Design review of the part built by this model. Coordinates are the model's own, in mm. Coordinates: 2 decimals unless noted, no trailing zeros. Order: outer loops, then holes, each group sorted by start corner. A loop starts at its lowest first (then second) coordinate and runs counter-clockwise, first axis right, second up. Notation, with made-up numbers: M -11.5,-9.5 L 4.5,-9.5 A18 cw 4.5,12.5 Z; hole C 6,84.25 d9. An arc over 180 degrees is marked long. Answer as a JSON object with one key per item and string values.
from build123d import *

# Parameters (mm, degrees)
SKETCH_1_R      = 12.5
SKETCH_1_R_2    = 2.1
SKETCH_1_R_3    = 1.6
EXTRUDE_1_DEPTH = 3
FILLET_2_R      = 7
FILLET_3_R      = 3
FILLET_4_R      = 0.5
CHAMFER_1_SIZE  = 2


with BuildPart() as part:
    # ｽｹｯﾁ1 → ﾎﾞｽ - 押し出し1 (new body)
    with BuildSketch(Plane.XY):
        with BuildLine():
            Line((-37.5, -3.5), (-16.63580476, -3.5))
            ThreePointArc((-16.63580476, -3.5), (-12.503868825, -11.517519889), (-4.852092963, -16.292857143))
            ThreePointArc((-4.852092963, -16.292857143), (0, -22.5), (4.852092963, -16.292857143))
            ThreePointArc((4.852092963, -16.292857143), (12.503868825, -11.517519889), (16.63580476, -3.5))
            Line((16.63580476, -3.5), (37.5, -3.5))
            ThreePointArc((37.5, -3.5), (41, 0), (37.5, 3.5))
            Line((37.5, 3.5), (20.5, 3.5))
            Line((20.5, 3.5), (20.5, 18))
            Line((20.5, 18), (14.5, 18))
            Line((14.5, 18), (14.5, 8.874119675))
            ThreePointArc((14.5, 8.874119675), (10.362687485, 13.476450129), (4.852092963, 16.292857143))
            ThreePointArc((4.852092963, 16.292857143), (0, 22.5), (-4.852092963, 16.292857143))
            ThreePointArc((-4.852092963, 16.292857143), (-10.362687485, 13.476450129), (-14.5, 8.874119675))
            Line((-14.5, 8.874119675), (-14.5, 18))
            Line((-14.5, 18), (-20.5, 18))
            Line((-20.5, 18), (-20.5, 3.5))
            Line((-20.5, 3.5), (-37.5, 3.5))
            ThreePointArc((-37.5, 3.5), (-41, 0), (-37.5, -3.5))
        make_face()
        Circle(SKETCH_1_R, mode=Mode.SUBTRACT)
        with Locations((0, 17.5)):
            Circle(SKETCH_1_R_2, mode=Mode.SUBTRACT)
        with Locations((-17.5, 0)):
            Circle(SKETCH_1_R_2, mode=Mode.SUBTRACT)
        with Locations((0, -17.5)):
            Circle(SKETCH_1_R_2, mode=Mode.SUBTRACT)
        with Locations((17.5, 0)):
            Circle(SKETCH_1_R_2, mode=Mode.SUBTRACT)
        with Locations((-27.5, 0)):
            Circle(SKETCH_1_R_3, mode=Mode.SUBTRACT)
        with Locations((-37.5, 0)):
            Circle(SKETCH_1_R_3, mode=Mode.SUBTRACT)
        with Locations((27.5, 0)):
            Circle(SKETCH_1_R_3, mode=Mode.SUBTRACT)
        with Locations((37.5, 0)):
            Circle(SKETCH_1_R_3, mode=Mode.SUBTRACT)
        with Locations((-17.5, 15)):
            Circle(SKETCH_1_R_3, mode=Mode.SUBTRACT)
        with Locations(Location((17.5, 15, 0), (0, 0, 180))):
            Circle(SKETCH_1_R_3, mode=Mode.SUBTRACT)
    extrude(amount=EXTRUDE_1_DEPTH)

    # ﾌｨﾚｯﾄ2
    fillet_2_edges = [part.edges().sort_by_distance(p)[0] for p in [
        (-4.852092963, 16.292857143, 1.5),
        (4.852092963, 16.292857143, 1.5),
        (16.63580476, -3.5, 1.5),
        (4.852092963, -16.292857143, 1.5),
        (-4.852092963, -16.292857143, 1.5),
        (-16.63580476, -3.5, 1.5),
    ]]
    fillet(fillet_2_edges, radius=FILLET_2_R)

    # ﾌｨﾚｯﾄ3
    fillet_3_edges = [part.edges().sort_by_distance(p)[0] for p in [
        (20.5, 18, 1.5),
        (14.5, 18, 1.5),
        (20.5, 3.5, 1.5),
        (-14.5, 18, 1.5),
        (-20.5, 18, 1.5),
        (-20.5, 3.5, 1.5),
    ]]
    fillet(fillet_3_edges, radius=FILLET_3_R - 0.0001)  # a hair under: the kernel refuses the full size

    # ﾌｨﾚｯﾄ4
    fillet_4_edges = [part.edges().sort_by_distance(p)[0] for p in [
        (14.5, 8.874119675, 1.5),
        (-14.5, 8.874119675, 1.5),
    ]]
    fillet(fillet_4_edges, radius=FILLET_4_R)

    # 面取り1
    chamfer_1_edges = [part.edges().sort_by_distance(p)[0] for p in [
        (-2.1, 17.5, 3),
        (-19.6, 0, 3),
        (-2.1, -17.5, 3),
        (15.4, 0, 3),
    ]]
    chamfer(chamfer_1_edges, length=CHAMFER_1_SIZE)


solid = part.part
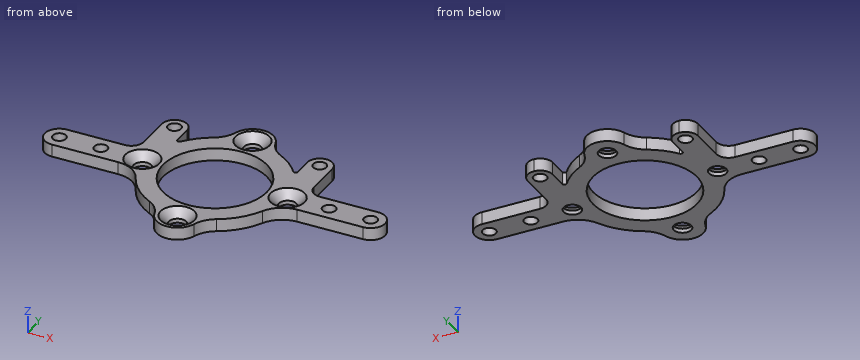
1) Add section D-D (y = 0). Count the separate pieces of the cut face and the enclosed holes in it, and give its area (3 significant figures).
Taken from the geometry:
{"separate pieces": "8", "enclosed holes": "0", "area": "99.4 mm2"}
2) Insertion check: pin 1 Ø1.5 at (x, z) = (-30.5, 2) entering from +Y; pin 2 Ø6.5 at (x, y) = (0, -17.5) entering from +Z; pin 3 Ø2.5 at (x, y) = (0, 17.5) entering from +Z; pin 4 Ø1.5 at (y, z) = (10, 1.5) entering from +X. Each pin has a flat end and moves straight along its axis. Give the tip position at first contact, or say it passes through.
Taken from the geometry:
{"pin 1": "stops at y = 3.5", "pin 2": "stops at z = 2.15", "pin 3": "passes through", "pin 4": "stops at x = 20.5"}
3) Add section C-C (x = 0). State the section outline as (y, z) points.
Taken from the geometry:
{"outline": "M -22.5,0 L -19.6,0 L -19.6,1 L -21.6,3 L -22.5,3 Z; M -15.4,0 L -12.5,0 L -12.5,3 L -13.4,3 L -15.4,1 Z; M 12.5,0 L 15.4,0 L 15.4,1 L 13.4,3 L 12.5,3 Z; M 19.6,0 L 22.5,0 L 22.5,3 L 21.6,3 L 19.6,1 Z"}
4) To check wall thickness, follow L1, parallel to Y at x = -37.5, z = 1.25; L2, parallel to Y at x = -17.5, z = 0.5; L3, parallel to Y at x = -17.5, z = 1.15. State the ranges of each line that lie inside material, in increasing order.
Taken from the geometry:
{"L1": "y = -3.5 to -1.6, 1.6 to 3.5", "L2": "y = -4.81 to -2.1, 2.1 to 13.4, 16.6 to 18", "L3": "y = -4.81 to -2.25, 2.25 to 13.4, 16.6 to 18"}
5) Add section A-A (x = 27.5). State the section outline as (y, z) points.
Taken from the geometry:
{"outline": "M -3.5,0 L -1.6,0 L -1.6,3 L -3.5,3 Z; M 1.6,0 L 3.5,0 L 3.5,3 L 1.6,3 Z"}
6) Add section B-B (y = -5). State the section outline as (x, z) points.
Taken from the geometry:
{"outline": "M -17.25,0 L -11.46,0 L -11.46,3 L -17.25,3 Z; M 11.46,0 L 17.25,0 L 17.25,3 L 11.46,3 Z"}
